from build123d import *

# Parameters (mm, degrees)
SKETCH_1_R               = 40
EXTRUDE_4_DEPTH          = 15
SKETCH_1_8_W             = 15
SKETCH_1_8_H             = 24
EXTRUDE_5_DEPTH          = 15
EXTRUDE_START            = 5
SKETCH_1_9_R             = 40
SKETCH_1_9_R_2           = 36
EXTRUDE_6_DEPTH          = 5
CUT_EXTRUDE_1_DEPTH      = 68.297845434
CUT_EXTRUDE_1_DEPTH_BACK = 68.297845434
SKETCH_2_R               = 7.5
FILLET_START             = -13
FILLET_1_DEPTH           = 26
CUT_EXTRUDE_2_DEPTH      = 83.861329943
CUT_EXTRUDE_2_DEPTH_BACK = 83.861329943
SKETCH_3_W               = 1.548025895
SKETCH_3_H               = 5.100179719
SKETCH_4_R               = 1.5
CUT_EXTRUDE_3_DEPTH      = 5
EXTRUDE_8_DEPTH          = 5
SKETCH_5_4_R             = 1.4
CUT_EXTRUDE_4_DEPTH      = 5


with BuildPart() as part:
    # 스케치1 → 보스-돌출4 (new body)
    with BuildSketch(Plane.XY):
        Circle(SKETCH_1_R)
    extrude(amount=-EXTRUDE_4_DEPTH)

    # 스케치1<8> → 보스-돌출5 (add)
    with BuildSketch(Plane.XY):
        with Locations((-23.5, 0)):
            Rectangle(SKETCH_1_8_W, SKETCH_1_8_H)
        with Locations((23.5, 0)):
            Rectangle(SKETCH_1_8_W, SKETCH_1_8_H)
    extrude(amount=EXTRUDE_5_DEPTH)

    # 스케치1<9> → 보스-돌출6 (add)
    with BuildSketch(Plane.XY.offset(EXTRUDE_START)):
        Circle(SKETCH_1_9_R)
        Circle(SKETCH_1_9_R_2, mode=Mode.SUBTRACT)
    extrude(amount=-EXTRUDE_6_DEPTH)

    # 스케치2 → 컷-돌출1 (cut, two sides: drawn at the far end of the back side and taken through both)
    with BuildSketch(Plane.XZ.offset(12).offset(-CUT_EXTRUDE_1_DEPTH_BACK)):
        with Locations((-23.5, 15)):
            Circle(SKETCH_2_R)
        with Locations((23.5, 15)):
            Circle(SKETCH_2_R)
    extrude(amount=CUT_EXTRUDE_1_DEPTH + CUT_EXTRUDE_1_DEPTH_BACK, mode=Mode.SUBTRACT)

    # 필렛1: read off the stored shape, not the designer's step
    # 필렛1 outline → 필렛1 (cut)
    with BuildSketch(Plane(origin=(0, 0, 0), x_dir=(1, 0, 0), z_dir=(0, 1, 0)).offset(FILLET_START)):
        with BuildLine():
            Line((31, -15), (31, -11.535898385))
            ThreePointArc((31, -11.535898385), (30.690007032, -11.925640266), (30.240506329, -11.711295935))
            ThreePointArc((30.240506329, -11.711295935), (30.807660278, -13.312368149), (31, -15))
        make_face()
        with BuildLine():
            ThreePointArc((16, -15), (16.192339722, -13.312368149), (16.759493671, -11.711295935))
            ThreePointArc((16.759493671, -11.711295935), (16.309992968, -11.925640266), (16, -11.535898385))
            Line((16, -11.535898385), (16, -15))
        make_face()
        with BuildLine():
            Line((-16, -15), (-16, -11.535898385))
            ThreePointArc((-16, -11.535898385), (-16.309992968, -11.925640266), (-16.759493671, -11.711295935))
            ThreePointArc((-16.759493671, -11.711295935), (-16.192339722, -13.312368149), (-16, -15))
        make_face()
        with BuildLine():
            ThreePointArc((-31, -15), (-30.807660278, -13.312368149), (-30.240506329, -11.711295935))
            ThreePointArc((-30.240506329, -11.711295935), (-30.690007032, -11.925640266), (-31, -11.535898385))
            Line((-31, -11.535898385), (-31, -15))
        make_face()
    extrude(amount=FILLET_1_DEPTH, mode=Mode.SUBTRACT)

    # 스케치3 → 컷-돌출2 (cut, two sides: drawn at the far end of the back side and taken through both)
    with BuildSketch(Plane(origin=(31, 0, 0), x_dir=(0, 0, -1), z_dir=(1, 0, 0)).offset(-CUT_EXTRUDE_2_DEPTH_BACK)):
        with Locations((-6.14855499, 0.540949065)):
            Rectangle(SKETCH_3_W, SKETCH_3_H)
    extrude(amount=CUT_EXTRUDE_2_DEPTH + CUT_EXTRUDE_2_DEPTH_BACK, mode=Mode.SUBTRACT)

    # 스케치4 → 컷-돌출3 (cut)
    with BuildSketch(Plane.XY):
        with Locations((7.5, 15)):
            Circle(SKETCH_4_R)
        with Locations((7.5, -15)):
            Circle(SKETCH_4_R)
    extrude(amount=-CUT_EXTRUDE_3_DEPTH, mode=Mode.SUBTRACT)

    # 스케치5 → 보스-돌출8 (add)
    with BuildSketch(Plane.XY):
        with BuildLine():
            Line((7.5, 15.1), (7.5, 15))
            Line((7.5, 15), (7.5, 13.5))
            ThreePointArc((7.5, 13.5), (8.560660172, 13.939339828), (9, 15))
            ThreePointArc((9, 15), (8.933057899, 15.443108405), (8.738206588, 15.846666667))
            ThreePointArc((8.738206588, 15.846666667), (8.222956891, 15.301111626), (7.5, 15.1))
        make_face()
        with BuildLine():
            Line((7.5, 13.5), (7.5, 15))
            Line((7.5, 15), (7.5, 15.1))
            ThreePointArc((7.5, 15.1), (6.777043109, 15.301111626), (6.261793412, 15.846666667))
            ThreePointArc((6.261793412, 15.846666667), (6.173350084, 14.3), (7.5, 13.5))
        make_face()
        with BuildLine():
            ThreePointArc((6.261793412, 15.846666667), (6.777043109, 15.301111626), (7.5, 15.1))
            Line((7.5, 15.1), (7.5, 16.5))
            ThreePointArc((7.5, 16.5), (6.8, 16.326649916), (6.261793412, 15.846666667))
        make_face()
        with BuildLine():
            Line((7.5, 16.5), (7.5, 15.1))
            ThreePointArc((7.5, 15.1), (8.222956891, 15.301111626), (8.738206588, 15.846666667))
            ThreePointArc((8.738206588, 15.846666667), (8.2, 16.326649916), (7.5, 16.5))
        make_face()
        with BuildLine():
            ThreePointArc((9, -15), (8.560660172, -13.939339828), (7.5, -13.5))
            Line((7.5, -13.5), (7.5, -15))
            Line((7.5, -15), (7.5, -15.1))
            ThreePointArc((7.5, -15.1), (8.222956891, -15.301111626), (8.738206588, -15.846666667))
            ThreePointArc((8.738206588, -15.846666667), (8.933057899, -15.443108405), (9, -15))
        make_face()
        with BuildLine():
            Line((7.5, -15), (7.5, -13.5))
            ThreePointArc((7.5, -13.5), (6.173350084, -14.3), (6.261793412, -15.846666667))
            ThreePointArc((6.261793412, -15.846666667), (6.777043109, -15.301111626), (7.5, -15.1))
            Line((7.5, -15.1), (7.5, -15))
        make_face()
        with BuildLine():
            ThreePointArc((7.5, -15.1), (6.777043109, -15.301111626), (6.261793412, -15.846666667))
            ThreePointArc((6.261793412, -15.846666667), (6.8, -16.326649916), (7.5, -16.5))
            Line((7.5, -16.5), (7.5, -15.1))
        make_face()
        with BuildLine():
            ThreePointArc((8.738206588, -15.846666667), (8.222956891, -15.301111626), (7.5, -15.1))
            Line((7.5, -15.1), (7.5, -16.5))
            ThreePointArc((7.5, -16.5), (8.2, -16.326649916), (8.738206588, -15.846666667))
        make_face()
    extrude(amount=-EXTRUDE_8_DEPTH)

    # 스케치5<4> → 컷-돌출4 (cut)
    with BuildSketch(Plane.XY):
        with Locations((7.5, 16.5)):
            Circle(SKETCH_5_4_R)
        with Locations((7.5, -16.5)):
            Circle(SKETCH_5_4_R)
    extrude(amount=-CUT_EXTRUDE_4_DEPTH, mode=Mode.SUBTRACT)


solid = part.part
Source: CAD feature listing. Evaluate the final solid. Frame: model axes, mm. A direction names the side the tool comes from. Give positions to 0.01 mm unless a question says otherwise; leave off trailing zeros. Write each loop counter-clockwise with the first axis right and the second up, starting at its lowest first coordinate (ties: lowest second). Pieces come first, ordered by that corner, then holes. Notation, with made-up numbers: (35, 9.25) -> (80, 9.25) arc R33 ccw to (80, 38.25) -> close; hole circle Ø10 at (-15.5, -35.75). An arc over 180 degrees is marked (long way). Return JSON: item names as keys, results as strings. Group by question number.
1. Section D-D, the plane z = -1.75. Output: boundary loops of the cut face in (x, y).
2. Pin query (flat end, axial travel): pin 1 Ø8 at (x, y) = (11, 11.5) entering from +Z; pin 2 Ø1 at (x, y) = (-27.5, 22.5) entering from +Z; pin 3 Ø2 at (x, z) = (12.5, -8.5) entering from -Y. Return the tip coordinate at first contact, or that it passes through.
3. Section B-B, the plane x = 7.5. Output: boundary loops of the cut face in (y, z).
4. Section A-A, the plane y = 0. Output: boundary loops of the cut face in (x, z).
5. Section C-C, the plane y = 33. Output: boundary loops of the cut face in (x, z).
6. Material intervals for line 1 (X direction, y = -8.5, z = 6.25); line 2 (Y direction, x = 7.5, z = -3.8); line 3 (X direction, y = -10, z = 0.25), sorted ascending. Write a range as from..to.
7. Mould query, pull axis X, two halves, no side actions, for faces 1 (the face through (-24, 1, 5.375)), 2 (the face through (-8.67, -39.05, -4.86)), 3 (the face through (7, -16, -5)). Classes: +X half, -X half, draft (parallel to the pull), parting line (faces both ways), or undercut.
8. Access query for faces 4 (the face through (23.4, 0.2, 7.5)), 5 (the face through (23, 1, 5.375)), 6 (the face through (6.47, -15.55, -2.46)). Directions: +Z, -Z, +X, -X, +Y, -Y. A direction counts if a zero-diameter tool reaches every point of the face in a straight line with its end or side. Return the directions, or none.
Determined:
{
 "1": {"outline": "circle Ø80 at (0, 0); hole circle Ø2.8 at (7.5, -16.5); hole circle Ø2.8 at (7.5, 16.5)"},
 "2": {"pin 1": "stops at z = 0", "pin 2": "stops at z = 5", "pin 3": "stops at y = -38.31"},
 "3": {"outline": "(-39.29, -15) -> (39.29, -15) -> (39.29, 5) -> (35.21, 5) -> (35.21, 0) -> (17.9, 0) -> (17.9, -5) -> (15.1, -5) -> (15.1, 0) -> (-15.1, 0) -> (-15.1, -5) -> (-17.9, -5) -> (-17.9, 0) -> (-35.21, 0) -> (-35.21, 5) -> (-39.29, 5) -> close"},
 "4": {"outline": "(-40, -15) -> (40, -15) -> (40, 5) -> (36, 5) -> (36, 0) -> (31, 0) -> (31, 5.37) -> (16, 5.37) -> (16, 0) -> (-16, 0) -> (-16, 5.37) -> (-31, 5.37) -> (-31, 0) -> (-36, 0) -> (-36, 5) -> (-40, 5) -> close; (-31, 6.92) -> (-16, 6.92) -> (-16, 11.54) arc R0.4 ccw to (-16.76, 11.71) arc R7.5 cw to (-30.24, 11.71) arc R0.4 ccw to (-31, 11.54) -> close; (16, 6.92) -> (31, 6.92) -> (31, 11.54) arc R0.4 ccw to (30.24, 11.71) arc R7.5 cw to (16.76, 11.71) arc R0.4 ccw to (16, 11.54) -> close"},
 "5": {"outline": "(-22.61, -15) -> (22.61, -15) -> (22.61, 5) -> (14.39, 5) -> (14.39, 0) -> (-14.39, 0) -> (-14.39, 5) -> (-22.61, 5) -> close"},
 "6": {"line 1": "x = -31..-16, 16..31", "line 2": "y = -39.29..-17.9, -15.1..15.1, 17.9..39.29", "line 3": "x = -38.73..-34.58, -31..-16, 16..31, 34.58..38.73"},
 "7": {"face 1": "draft", "face 2": "parting line", "face 3": "undercut"},
 "8": {"face 4": "+Z, +Y, -Y", "face 5": "+X, -X", "face 6": "+Z"}
}
